Read the model definition and answer for the solid it produces. Units are mm, in the model's axes. Round coordinates to 2 decimals unless told otherwise and drop trailing zeros. Loops run counter-clockwise (first coordinate to the right, second up) from the corner with the lowest first, then second, coordinate; pieces in that order, holes last. Notation, with made-up numbers: (28, 54.5) - (78, 54.5) arc R13 ccw to (78, 79.5) - close; hole circle Ø6 at (3, 60). An arc over 180 degrees is marked (long way). Use CSV: the item, a comma, the result in double quotes. Start each with the question number.
1. Find section C-C (y = -13.5). State how many separate pieces and enclosed holes the cut face has, and give its area (3 significant figures).
2. Consider line 1 along Y through (x, z) = (12, 2.15); line 2 along X through (y, z) = (10, 1.4); line 3 along Y through (x, z) = (0, 2.2) (3 decimals). Determine where each line is inside the solid, lowest interval first.
3. Find section A-A (x = 9). Give the vertices of the cut face in (y, z).
4. Find section B-B (y = 0). Give the vertices of the cut face in (x, z) (3 decimals).
Autodesk Inventor part; units mm, degrees
ref_plane "YZ Plane" through (0, 0, 0) normal (1, 0, 0) x (0, 1, 0)
ref_plane "XZ Plane" through (0, 0, 0) normal (0, 1, 0) x (-1, 0, 0)
ref_plane "XY Plane" through (0, 0, 0) normal (0, 0, 1) x (1, 0, 0)
sketch "Sketch1" plane through (0, 0, 0) normal (0, 0, 1) x (1, 0, 0)
  circle A0 centre (-5.816, 5.816) radius 1.25
  circle A1 centre (5.816, 5.816) radius 1.25
  circle A2 centre (5.816, -5.816) radius 1.25
  circle A3 centre (-5.816, -5.816) radius 1.25
  circle A4 centre (0, 0) radius 11
  circle A5 centre (0, 0) radius 5.125
  circle A6 centre (30.8333, 0) radius 6.096
  circle A7 centre (-30.8333, 0) radius 6.096
  line L0 (30.8333, 0) -> (-30.8333, 0) construction
  line L1 (-60, 25) -> (60, 25)
  line L2 (60, 25) -> (60, -25)
  line L3 (60, -25) -> (-60, -25)
  line L4 (-60, -25) -> (-60, 25)
  line L5 (0, 25) -> (0, -25) construction
  point P0 (0, 0)
  dimension "d9" = 2.5
  dimension "d10" = 2.5
  dimension "d11" = 2.5
  dimension "d12" = 2.5
  dimension "d33" = 120
  dimension "d34" = 50
extrude "Extrusion1" add sketch "Sketch1" along normal blind 3 contours A4 | L1 L2 L3 L4
sketch "Sketch2" plane through (0, 0, 3) normal (0, 0, 1) x (1, 0, 0)
  line L0 (42.3333, -16.6667) -> (39.3333, -16.6667)
  line L1 (39.3333, -16.6667) -> (39.3333, -8.65)
  line L2 (39.3333, -8.65) -> (42.3333, -8.65)
  line L3 (42.3333, -8.65) -> (42.3333, -16.6667)
  line L4 (39.3333, 3.35) -> (42.3333, 3.35)
  line L5 (42.3333, 3.35) -> (42.3333, -3.35)
  line L6 (42.3333, -3.35) -> (39.3333, -3.35)
  line L7 (39.3333, -3.35) -> (39.3333, 3.35)
  line L8 (42.3333, 8.65) -> (39.3333, 8.65)
  line L9 (39.3333, 8.65) -> (39.3333, 16.6667)
  line L10 (39.3333, 16.6667) -> (42.3333, 16.6667)
  line L11 (42.3333, 16.6667) -> (42.3333, 8.65)
  line L12 (-39.3333, -16.6667) -> (-42.3333, -16.6667)
  line L13 (-42.3333, -16.6667) -> (-42.3333, -8.65)
  line L14 (-42.3333, -8.65) -> (-39.3333, -8.65)
  line L15 (-39.3333, -8.65) -> (-39.3333, -16.6667)
  line L16 (-42.3333, 3.35) -> (-39.3333, 3.35)
  line L17 (-39.3333, 3.35) -> (-39.3333, -3.35)
  line L18 (-39.3333, -3.35) -> (-42.3333, -3.35)
  line L19 (-42.3333, -3.35) -> (-42.3333, 3.35)
  line L20 (-39.3333, 8.65) -> (-42.3333, 8.65)
  line L21 (-42.3333, 8.65) -> (-42.3333, 16.6667)
  line L22 (-42.3333, 16.6667) -> (-39.3333, 16.6667)
  line L23 (-39.3333, 16.6667) -> (-39.3333, 8.65)
  line L24 (19.3333, -5) -> (22.3333, -5)
  line L25 (22.3333, -5) -> (22.3333, -15)
  line L26 (22.3333, -15) -> (19.3333, -15)
  line L27 (19.3333, -15) -> (19.3333, -5)
  line L28 (22.3333, 5) -> (19.3333, 5)
  line L29 (19.3333, 5) -> (19.3333, 15)
  line L30 (19.3333, 15) -> (22.3333, 15)
  line L31 (22.3333, 15) -> (22.3333, 5)
  circle A0 centre (40.8333, 6) radius 1.4
  circle A1 centre (40.8333, -6) radius 1.4
  circle A2 centre (-40.8333, 6) radius 1.4
  circle A3 centre (-40.8333, -6) radius 1.4
  line L32 (33.4833, 12) -> (33.4833, 15)
  line L33 (33.4833, 15) -> (35.9333, 15)
  line L34 (35.9333, 15) -> (35.9333, 12)
  line L35 (35.9333, 12) -> (33.4833, 12)
  line L36 (28.1833, 15) -> (28.1833, 12)
  line L37 (28.1833, 12) -> (25.7333, 12)
  line L38 (25.7333, 12) -> (25.7333, 15)
  line L39 (25.7333, 15) -> (28.1833, 15)
  line L40 (-25.1833, 12) -> (-25.1833, 15)
  line L41 (-25.1833, 15) -> (-20.9333, 15)
  line L42 (-20.9333, 15) -> (-20.9333, 12)
  line L43 (-20.9333, 12) -> (-25.1833, 12)
  line L44 (-30.4833, 15) -> (-30.4833, 12)
  line L45 (-30.4833, 12) -> (-34.7333, 12)
  line L46 (-34.7333, 12) -> (-34.7333, 15)
  line L47 (-34.7333, 15) -> (-30.4833, 15)
  line L48 (12.8, 12) -> (-6.8, 12)
  line L49 (-6.8, 12) -> (-6.8, 15)
  line L50 (-6.8, 15) -> (12.8, 15)
  line L51 (12.8, 15) -> (12.8, 12)
  line L52 (-16.3333, -5) -> (-13.3333, -5)
  line L53 (-13.3333, -5) -> (-13.3333, -15)
  line L54 (-13.3333, -15) -> (-16.3333, -15)
  line L55 (-16.3333, -15) -> (-16.3333, -5)
  line L56 (-13.3333, 5) -> (-16.3333, 5)
  line L57 (-16.3333, 5) -> (-16.3333, 15)
  line L58 (-16.3333, 15) -> (-13.3333, 15)
  line L59 (-13.3333, 15) -> (-13.3333, 5)
  line L60 (-30.4833, -12) -> (-30.4833, -15)
  line L61 (-30.4833, -15) -> (-34.7333, -15)
  line L62 (-34.7333, -15) -> (-34.7333, -12)
  line L63 (-34.7333, -12) -> (-30.4833, -12)
  line L64 (-25.1833, -15) -> (-25.1833, -12)
  line L65 (-25.1833, -12) -> (-20.9333, -12)
  line L66 (-20.9333, -12) -> (-20.9333, -15)
  line L67 (-20.9333, -15) -> (-25.1833, -15)
  line L68 (28.1833, -12) -> (28.1833, -15)
  line L69 (28.1833, -15) -> (25.7333, -15)
  line L70 (25.7333, -15) -> (25.7333, -12)
  line L71 (25.7333, -12) -> (28.1833, -12)
  line L72 (33.4833, -15) -> (33.4833, -12)
  line L73 (33.4833, -12) -> (35.9333, -12)
  line L74 (35.9333, -12) -> (35.9333, -15)
  line L75 (35.9333, -15) -> (33.4833, -15)
  line L76 (-6.8, -12) -> (12.8, -12)
  line L77 (12.8, -12) -> (12.8, -15)
  line L78 (12.8, -15) -> (-6.8, -15)
  line L79 (-6.8, -15) -> (-6.8, -12)
  circle A4 centre (-27.8333, 13.5) radius 1.4
  circle A5 centre (-27.8333, -13.5) radius 1.4
  circle A6 centre (30.8333, -13.5) radius 1.4
  circle A7 centre (30.8333, 13.5) radius 1.4
  point P0 (0, 0)
  dimension "d35" = 2.8
  dimension "d36" = 2.8
  dimension "d37" = 5.3
  dimension "d38" = 2.65
  dimension "d39" = 2.65
  dimension "d40" = 2.8
  dimension "d41" = 2.8
  dimension "d42" = 2.65
  dimension "d43" = 2.65
  dimension "d44" = 2.8
  dimension "d45" = 5.3
  dimension "d46" = 2.65
  dimension "d47" = 2.8
  dimension "d48" = 2.8
  dimension "d49" = 5.3
  dimension "d50" = 2.65
  dimension "d51" = 2.8
extrude "Extrusion2" cut sketch "Sketch2" against normal blind 3
equation "\"d38\" = 0.5 * d37"
equation "\"d39\" = d38"
equation "\"d42\" = d38"
equation "\"d43\" = d42"
equation "\"d46\" = 0.5 * d45"
equation "\"d50\" = 0.5 * d49"
properties part number "Camera-Holder_Front"
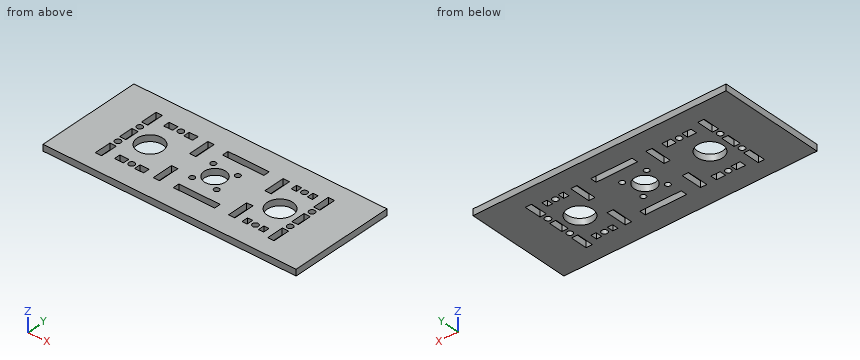
Filled sheet:
1,separate pieces,"12"
1,enclosed holes,"0"
1,area,"208 mm²"
2,line 1,"y = -25 to -15, -12 to 12, 15 to 25"
2,line 2,"x = -60 to -42.33, -39.33 to -16.33, -13.33 to 19.33, 22.33 to 39.33, 42.33 to 60"
2,line 3,"y = -25 to -15, -12 to -5.125, 5.125 to 12, 15 to 25"
3,outline,"(-25, 0) - (-15, 0) - (-15, 3) - (-25, 3) - close; (-12, 0) - (12, 0) - (12, 3) - (-12, 3) - close; (15, 0) - (25, 0) - (25, 3) - (15, 3) - close"
4,outline,"(-60, 0) - (-42.333, 0) - (-42.333, 3) - (-60, 3) - close; (-39.333, 0) - (-36.929, 0) - (-36.929, 3) - (-39.333, 3) - close; (-24.737, 0) - (-5.125, 0) - (-5.125, 3) - (-24.737, 3) - close; (5.125, 0) - (24.737, 0) - (24.737, 3) - (5.125, 3) - close; (36.929, 0) - (39.333, 0) - (39.333, 3) - (36.929, 3) - close; (42.333, 0) - (60, 0) - (60, 3) - (42.333, 3) - close"
